Part model, mm, in its own coordinate system. A direction names the side the tool comes from. Coordinates: 2 decimals unless noted, no trailing zeros. Loops run counter-clockwise (first coordinate to the right, second up) from the corner with the lowest first, then second, coordinate; pieces in that order, holes last. Notation, with made-up numbers: (-11.75, -40) - (21.25, -40) arc R29 ccw to (21.25, -16) - close; hole circle Ø6 at (-6, 70). An arc over 180 degrees is marked (long way). Use a Markdown table: item, result. Add a question column.
1. Drop a flat-ended pin along its axis: pin 1 (1.5 mm diameter, centred on y = 3, z = 7, fed in from +X). Give the stop position or say it passes through.
2. Band-saw the part on D-D, the plane z = 5. Give the cut face in (x, y).
3. Wall check: probe 1 along Z at (x, y) = (34.5, 3.75); probe 2 along X at (y, z) = (1.5, -4.25); probe 3 along X at (y, z) = (0.75, 0.5). Give the ranges that are in metal, low to high. Write a range as [from, to].
4. Pull direction Z, two halves, no side cores. Call faces 1 (the cylindrical face through (46, 2, 0)), 2 (the cylindrical face through (36, 2, 0)), 3 (the flat face through (32, 2, -6)), 4 (the flat face through (19, 2, -10)): pulls with the +Z half, pulls with the -Z half, needs draft (parallel to the pull), parting line crosses it, or undercut.
5. Band-saw the part on C-C, the plane z = -1.5. Give the cut face in (x, y).
6. Band-saw the part on B-B, the plane y = 0.85. Give the cut face in (x, z).
7. Band-saw the part on A-A, the plane x = 31.5. Give the cut face in (y, z), plus the area to 3 significant figures.
8. 3-axis set-ups, long thin cutter, end or side, ignore diameter. For faces 5 (the cylindrical face through (-6.948, 1.972, 0.22)), 6 (the cylindrical face through (5.416, 1.972, 5.449)): which of +Z, -Z, +X, -X, +Y, -Y reach the whole face in a straight line?
from build123d import *

# Parameters (mm, degrees)
SKETCH1_R           = 2
SKETCH1_R_2         = 3.05
BOSS_EXTRUDE1_DEPTH = 4


with BuildPart() as part:
    # Sketch1 → Boss-Extrude1 (new body)
    with BuildSketch(Plane(origin=(0, 0, 0), x_dir=(1, 0, 0), z_dir=(0, 1, 0))):
        with BuildLine():
            Line((3.05, 10), (36, 10))
            ThreePointArc((36, 10), (46, 0), (36, -10))
            Line((36, -10), (3.05, -10))
            ThreePointArc((3.05, -10), (-6.95, 0), (3.05, 10))
        make_face()
        with Locations(Location((42, 0, 0), (0, 0, 270))):
            Circle(SKETCH1_R, mode=Mode.SUBTRACT)
        with Locations(Location((0, 0, 0), (0, 0, 270))):
            Circle(SKETCH1_R_2, mode=Mode.SUBTRACT)
        with Locations(Location((20, 0, 0), (0, 0, 270))):
            Circle(SKETCH1_R_2, mode=Mode.SUBTRACT)
        with BuildLine():
            Line((26.308922253, -6), (37.101020514, -6))
            ThreePointArc((37.101020514, -6), (38.026840614, -5.377964473), (37.800874727, -4.285714286))
            ThreePointArc((37.800874727, -4.285714286), (36, 0), (37.800874727, 4.285714286))
            ThreePointArc((37.800874727, 4.285714286), (38.026840614, 5.377964473), (37.101020514, 6))
            Line((37.101020514, 6), (26.308922253, 6))
            ThreePointArc((26.308922253, 6), (25.408611748, 5.435248198), (25.525205203, 4.378881988))
            ThreePointArc((25.525205203, 4.378881988), (27.05, 0), (25.525205203, -4.378881988))
            ThreePointArc((25.525205203, -4.378881988), (25.408611748, -5.435248198), (26.308922253, -6))
        make_face(mode=Mode.SUBTRACT)
        with BuildLine():
            Line((6.308922253, 6), (13.691077747, 6))
            ThreePointArc((13.691077747, 6), (14.591388252, 5.435248198), (14.474794797, 4.378881988))
            ThreePointArc((14.474794797, 4.378881988), (12.95, 0), (14.474794797, -4.378881988))
            ThreePointArc((14.474794797, -4.378881988), (14.591388252, -5.435248198), (13.691077747, -6))
            Line((13.691077747, -6), (6.308922253, -6))
            ThreePointArc((6.308922253, -6), (5.408611748, -5.435248198), (5.525205203, -4.378881988))
            ThreePointArc((5.525205203, -4.378881988), (7.05, 0), (5.525205203, 4.378881988))
            ThreePointArc((5.525205203, 4.378881988), (5.408611748, 5.435248198), (6.308922253, 6))
        make_face(mode=Mode.SUBTRACT)
    extrude(amount=BOSS_EXTRUDE1_DEPTH)


solid = part.part
Geometry check:
| question | item | result |
|---|---|---|
| 1 | pin 1 | stops at x = 43.81 |
| 2 | outline | (-5.61, 0) - (5.31, 0) - (5.31, 4) - (-5.61, 4) - close; (14.69, 0) - (25.31, 0) - (25.31, 4) - (14.69, 4) - close; (38.1, 0) - (44.66, 0) - (44.66, 4) - (38.1, 4) - close |
| 3 | probe 1 | z = [-10, -6], [6, 10] |
| 3 | probe 2 | x = [-6, 5.62], [14.38, 25.62], [37.76, 45.05] |
| 3 | probe 3 | x = [-6.94, -3.01], [3.01, 7.03], [12.97, 16.99], [23.01, 27.03], [36.02, 40.06], [43.94, 45.99] |
| 4 | face 1 | parting line crosses it |
| 4 | face 2 | undercut |
| 4 | face 3 | undercut |
| 4 | face 4 | pulls with the -Z half |
| 5 | outline | (-6.84, 0) - (-2.66, 0) - (-2.66, 4) - (-6.84, 4) - close; (2.66, 0) - (6.89, 0) - (6.89, 4) - (2.66, 4) - close; (13.11, 0) - (17.34, 0) - (17.34, 4) - (13.11, 4) - close; (22.66, 0) - (26.89, 0) - (26.89, 4) - (22.66, 4) - close; (36.19, 0) - (40.68, 0) - (40.68, 4) - (36.19, 4) - close; (43.32, 0) - (45.89, 0) - (45.89, 4) - (43.32, 4) - close |
| 6 | outline | (3.05, -10) - (36, -10) arc R10 ccw to (36, 10) - (3.05, 10) arc R10 ccw to start; hole circle Ø6.1 at (0, 0); hole (5.53, -4.38) arc R1 ccw to (6.31, -6) - (13.69, -6) arc R1 ccw to (14.47, -4.38) arc R7.05 cw to (14.47, 4.38) arc R1 ccw to (13.69, 6) - (6.31, 6) arc R1 ccw to (5.53, 4.38) arc R7.05 cw to start; hole circle Ø6.1 at (20, 0); hole (25.53, -4.38) arc R1 ccw to (26.31, -6) - (37.1, -6) arc R1 ccw to (37.8, -4.29) arc R6 cw to (37.8, 4.29) arc R1 ccw to (37.1, 6) - (26.31, 6) arc R1 ccw to (25.53, 4.38) arc R7.05 cw to start; hole circle Ø4 at (42, 0) |
| 7 | outline | (0, -10) - (4, -10) - (4, -6) - (0, -6) - close; (0, 6) - (4, 6) - (4, 10) - (0, 10) - close |
| 7 | area | 32.0 mm^2 |
| 8 | face 5 | -X, +Y, -Y |
| 8 | face 6 | +Y, -Y |
